Could you check a few things on this model? Use its own coordinates, in mm. A direction names the side the tool comes from. Round coordinates to 2 decimals unless told otherwise and drop trailing zeros. Loops run counter-clockwise (first coordinate to the right, second up) from the corner with the lowest first, then second, coordinate; pieces in that order, holes last. Notation, with made-up numbers: (88, 45) -> (140, 45) arc R7 cw to (140, 50) -> close; hole circle Ø10 at (-35, 69). An arc over 180 degrees is marked (long way). One line per item, written item: value.
```python
from build123d import *

# Parameters (mm, degrees)
IZIM1_R                     = 1.89
Y_KSEKLIK_EKSTR_ZYON1_DEPTH = 48
Y_KSEKLIK_EKSTR_ZYON2_DEPTH = 2.5
Y_KSEKLIK_EKSTR_ZYON3_DEPTH = 1.5
Y_KSEKLIK_EKSTR_ZYON7_DEPTH = 1.5
Y_KSEKLIK_EKSTR_ZYON8_DEPTH = 0.5
IZIM6_4_R                   = 1.461469514
Y_KSEKLIK_EKSTR_ZYON9_DEPTH = 1
IZIM8_R                     = 1.032330659
KES_EKSTR_ZYON1_DEPTH       = 4


with BuildPart() as part:
    # izim1 → Y_kseklik-Ekstr_zyon1 (new body)
    with BuildSketch(Plane.XY):
        Circle(IZIM1_R)
    extrude(amount=Y_KSEKLIK_EKSTR_ZYON1_DEPTH)

    # izim2 → Y_kseklik-Ekstr_zyon2 (add, symmetric)
    with BuildSketch(Plane.XY.offset(23)):
        with BuildLine():
            Line((-2.329785398, 1.89), (0, 1.89))
            Line((0, 1.89), (0, -1.824067041))
            Line((0, -1.824067041), (-2.381759734, -1.824067041))
            ThreePointArc((-2.381759734, -1.824067041), (0.962995534, -2.841239096), (3, 0))
            ThreePointArc((3, 0), (1.002657421, 2.82748618), (-2.329785398, 1.89))
        make_face()
        with BuildLine():
            Line((0, -1.824067041), (0, 1.89))
            Line((0, 1.89), (-2.329785398, 1.89))
            ThreePointArc((-2.329785398, 1.89), (-2.999706299, 0.041977633), (-2.381759734, -1.824067041))
            Line((-2.381759734, -1.824067041), (0, -1.824067041))
        make_face()
    extrude(amount=Y_KSEKLIK_EKSTR_ZYON2_DEPTH, both=True)

    # izim2_3 → Y_kseklik-Ekstr_zyon3 (add, symmetric)
    with BuildSketch(Plane.XY.offset(23)):
        with BuildLine():
            ThreePointArc((-2.381759734, -1.824067041), (-2.999706299, 0.041977633), (-2.329785398, 1.89))
            Line((-2.329785398, 1.89), (-7.072158803, 1.89))
            Line((-7.072158803, 1.89), (-8.144317606, 0.03296648))
            Line((-8.144317606, 0.03296648), (-7.072158803, -1.824067041))
            Line((-7.072158803, -1.824067041), (-2.381759734, -1.824067041))
        make_face()
    extrude(amount=Y_KSEKLIK_EKSTR_ZYON3_DEPTH, both=True)

    # izim6 → Y_kseklik-Ekstr_zyon7 (add, symmetric)
    with BuildSketch(Plane.XY.offset(23)):
        with BuildLine():
            Line((9.765618481, 12.085389192), (-1.318138223, 1.362498594))
            ThreePointArc((-1.318138223, 1.362498594), (-1.362498594, -1.318138223), (1.318138223, -1.362498594))
            Line((1.318138223, -1.362498594), (12.401894927, 9.360392003))
            ThreePointArc((12.401894927, 9.360392003), (12.83161994, 9.988816416), (12.979469937, 10.735623759))
            Line((12.979469937, 10.735623759), (11.327344102, 10.094845982))
            ThreePointArc((11.327344102, 10.094845982), (10.455712089, 10.4793032), (10.840169306, 11.350935213))
            Line((10.840169306, 11.350935213), (12.492295142, 11.99171299))
            ThreePointArc((12.492295142, 11.99171299), (11.148847851, 12.617528805), (9.765618481, 12.085389192))
        make_face()
        with BuildLine():
            ThreePointArc((12.979469937, 10.735623759), (12.851229424, 11.408405718), (12.492295142, 11.99171299))
            Line((12.492295142, 11.99171299), (10.840169306, 11.350935213))
            ThreePointArc((10.840169306, 11.350935213), (10.455712089, 10.4793032), (11.327344102, 10.094845982))
            Line((11.327344102, 10.094845982), (12.979469937, 10.735623759))
        make_face()
    extrude(amount=Y_KSEKLIK_EKSTR_ZYON7_DEPTH, both=True)

    # izim6_3 → Y_kseklik-Ekstr_zyon8 (add, symmetric)
    with BuildSketch(Plane.XY.offset(23)):
        with BuildLine():
            Line((10.840169306, 11.350935213), (16.272383955, 13.457822202))
            ThreePointArc((16.272383955, 13.457822202), (17.144015968, 13.073364985), (16.75955875, 12.201732972))
            Line((16.75955875, 12.201732972), (11.327344102, 10.094845982))
            ThreePointArc((11.327344102, 10.094845982), (10.455712089, 10.4793032), (10.840169306, 11.350935213))
        make_face()
    extrude(amount=Y_KSEKLIK_EKSTR_ZYON8_DEPTH, both=True)

    # izim6_4 → Y_kseklik-Ekstr_zyon9 (add, symmetric)
    with BuildSketch(Plane.XY.offset(23)):
        with Locations((16.515971352, 12.829777587)):
            Circle(IZIM6_4_R)
    extrude(amount=Y_KSEKLIK_EKSTR_ZYON9_DEPTH, both=True)

    # izim8 → Kes-Ekstr_zyon1 (cut)
    with BuildSketch(Plane.XY.offset(24.5)):
        with Locations((-6, 0.03296648)):
            Circle(IZIM8_R)
    extrude(amount=-KES_EKSTR_ZYON1_DEPTH, mode=Mode.SUBTRACT)


solid = part.part
```
(1) Imagine slicing it at B-B on z = 11. Write out the boundary of the cut face in (x, y), then the cut area to 3 significant figures.
Results below:
outline: circle Ø3.78 at (0, 0)
area: 11.2 mm²
(2) Imagine slicing it at C-C on y = 8.5. Write out the boundary of the cut face in (x, z), then the cut area to 3 significant figures.
Results below:
outline: (6.06, 21.5) -> (11.51, 21.5) -> (11.51, 24.5) -> (6.06, 24.5) -> close
area: 16.4 mm²
(3) Please list where these lines run through material, in increasing order: L1, parallel to Y at x = -6, z = 22.6; L2, parallel to Z at x = 12.25, y = 10.25; L3, parallel to X at y = -1, z = 44.
Results below:
L1: y = -1.82 to -1, 1.07 to 1.89
L2: z = 21.5 to 24.5
L3: x = -1.6 to 1.6
(4) On a 3-axis mill with a long thin cutter (end or side, diameter ignored), from which of +Z, -Z, +X, -X, +Y, -Y can I reach the whole of each face in a straight line? I mean faces 4 (the face through (16, 13, 24)), 5 (the face through (-5, 1.89, 23)), 6 (the face through (-0.41, -1.845, 10.106)), 7 (the face through (14.28, 11.24, 23.01)). Say none if no direction works.
Results below:
face 4: +Z, +X, +Y, -Y
face 5: +Z, -Z, -X, +Y
face 6: -Z
face 7: +Z, -Z, -Y
(5) Imagine slicing it at D-D on x = 6.75. Write out the boundary of the cut face in (y, z).
Results below:
outline: (3.89, 21.5) -> (9.17, 21.5) -> (9.17, 24.5) -> (3.89, 24.5) -> close
(6) For pin 1 Ø1.1 at (x, y) = (14.5, 11.5) entering from +Z; pin 2 Ø6 at (x, y) = (9.5, 6) entering from -Z; pin 3 Ø4 at (x, y) = (-6, -0.5) entering from +Z, each with a flat end and sliding along its axis, tell me the tip position at first contact or that it passes through.
Results below:
pin 1: stops at z = 23.5
pin 2: stops at z = 21.5
pin 3: stops at z = 24.5
(7) Imagine slicing it at A-A on x = -6. Write out the boundary of the cut face in (y, z).
Results below:
outline: (-1.82, 21.5) -> (-1, 21.5) -> (-1, 24.5) -> (-1.82, 24.5) -> close; (1.07, 21.5) -> (1.89, 21.5) -> (1.89, 24.5) -> (1.07, 24.5) -> close
(8) We'd pull the mould along X, two halves only. Please class faces 1 (the face through (-5, -1.824, 23)), 2 (the face through (13.8, 12.5, 23)), 3 (the face through (-7.601, 0.974, 23.021)): +X half, -X half, draft (parallel to the pull), parting line (faces both ways), or undercut.
Results below:
face 1: draft
face 2: undercut
face 3: -X half
